Input: part model. Units: mm. Frame: model coordinates. Face numbers are marked on the shaded views. Coordinates: 2 decimals unless noted, no trailing zeros. Write each loop counter-clockwise with the first axis right and the second up, starting at its lowest first coordinate (ties: lowest second). Pieces come first, ordered by that corner, then holes. Notation, with made-up numbers: (-35, -36.75) - (-3, -36.75) arc R22 ccw to (-3, -8.75) - close; hole circle Ø11 at (64.5, -35.75). An arc over 180 degrees is marked (long way). Put each result on its own line as item: value. Start each with the question number.
1. Line query: line 1 (X direction, y = 0, z = 54); line 2 (Y direction, x = 47, z = 56); line 3 (X direction, y = 0, z = 91). Output: solid intervals per line, ascending.
2. Pull-direction query (Z, two-part tool) for the marked faces 1, 2, 3 and 4; classes: released by +Z, released by -Z, zero draft, split by the parting line, or undercut.
3. Pin query (flat end, axial travel): pin 1 (12 mm diameter, centred on x = 97.5, y = 19, fed in from -Z); pin 2 (1 mm diameter, centred on y = 16, z = 103, fed in from -X); pin 3 (8 mm diameter, centred on y = -33.5, z = 90.5, fed in from +X). Return the tip coordinate at first contact, or that it passes through.
4. Cut plane C-C, the plane z = 53. Return loops of the section in (x, y), and give its area (3 significant figures).
5. Cut plane B-B, the plane y = -3. Count the separate pieces of the cut face and the enclosed holes in it, and give its area (3 significant figures).
6. Cut plane A-A, the plane z = 74.5. Return loops of the section in (x, y), and give its area (3 significant figures).
from build123d import *

# Parameters (mm, degrees)
F2_R     = 37.958364699
F3_DEPTH = 25.399999693


with BuildPart() as f1:
    # F0 (on Front) → F1 (revolve)
    with BuildSketch(Plane.XZ):
        Polygon((115.5123189092, 116.3347512484), (83.8526785374, 105.7259817888), (83.8526785374, 41.3565523922), (115.743175149, 51.0456599295), align=None)
    revolve(axis=Axis((60.2732487023, 0, 87.5743832439), (0, 0, -1)))

    # F2 (on Right) → F3 (cut)
    with BuildSketch(Plane.YZ):
        with Locations((-11.3635012621, 75.3479318831)):
            Circle(F2_R)
    extrude(amount=F3_DEPTH, mode=Mode.SUBTRACT)


solid = f1.part
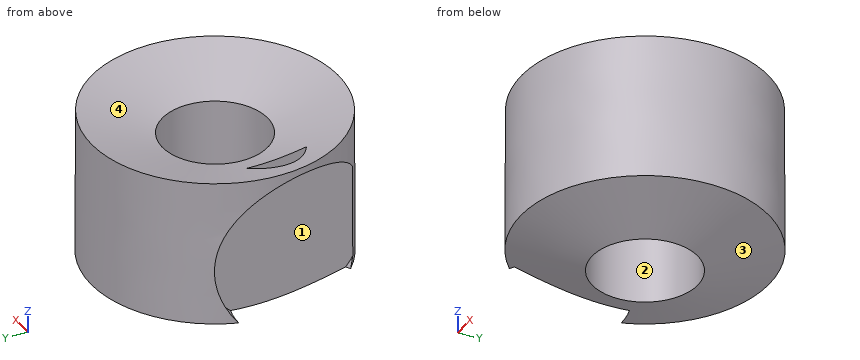
Report:
1. line 1: x = 25.4 to 36.69, 83.85 to 115.73
1. line 2: y = -53.84 to -19.49, 19.49 to 53.84
1. line 3: x = 25.4 to 36.69, 83.85 to 115.6
2. face 1: undercut
2. face 2: zero draft
2. face 3: released by -Z
2. face 4: released by +Z
3. pin 1: stops at z = 45.07
3. pin 2: stops at x = 7.2
3. pin 3: stops at x = 107.08
4. outline: (8.28, 19.32) - (25.4, 19.32) - (25.4, -42.05) - (24.1, -42.05) arc R55.46 ccw (long way) to start; hole circle Ø47.16 at (60.27, 0)
4. area: 6,920 mm^2
5. separate pieces: 3
5. enclosed holes: 0
5. area: 2,830 mm^2
6. outline: (11.68, 26.59) - (25.4, 26.59) - (25.4, -43.03) arc R55.39 ccw (long way) to start; hole circle Ø47.16 at (60.27, 0)
6. area: 6,790 mm^2
